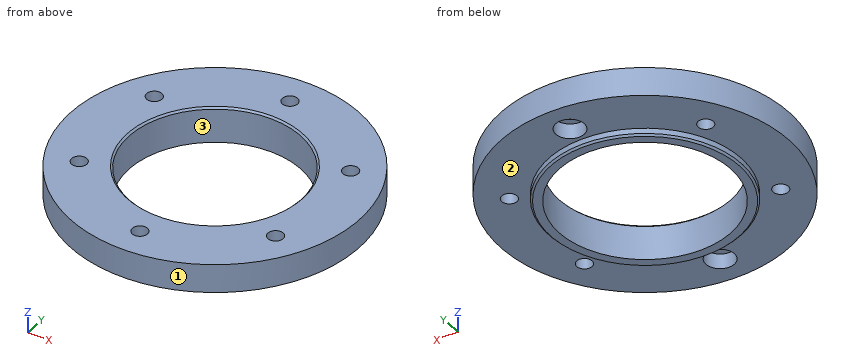
Autodesk Inventor part; units mm, degrees
ref_plane "YZ Plane" through (0, 0, 0) normal (1, 0, 0) x (0, 1, 0)
ref_plane "XZ Plane" through (0, 0, 0) normal (0, 1, 0) x (-1, 0, 0)
ref_plane "XY Plane" through (0, 0, 0) normal (0, 0, 1) x (1, 0, 0)
sketch "スケッチ2" plane through (0, 0, 0) normal (1, 0, 0) x (0, 1, 0)
  line L0 (24.1, 0) -> (24.1, -10)
  line L1 (40.5, 0) -> (40.5, -8)
  line L2 (40.5, 0) -> (24.1, 0)
  line L3 (24.1, 0) -> (59, 0)
  line L4 (24.1, -10) -> (27, -10)
  line L5 (0, -12) -> (0, 2)
  line L6 (27, -10) -> (27, -8)
  line L7 (27, -8) -> (40.5, -8)
  point P0 (0, 0)
  dimension "d40" = 24.1
  dimension "d41" = 8
  dimension "d42" = 40.5
  dimension "d43" = 27
  dimension "d44" = 2
revolve "回転1" add sketch "スケッチ2" angle 360 about axis through (0, 0, -10) along (0, 0, 1)
sketch "スケッチ4" plane through (0, 0, 0) normal (0, 0, 1) x (1, 0, 0)
  point P0 (0, 0)
  point P1 (0, 32)
  point P2 (-27.7128, 16)
  point P3 (-27.7128, -16)
  point P4 (0, -32)
  point P5 (27.7128, -16)
  point P6 (27.7128, 16)
  dimension "d11" = 32
  dimension "d14" = 360
hole "穴1" at (0, 32, 0) at (-27.7128, 16, 0) at (-27.7128, -16, 0) at (0, -32, 0) at (27.7128, -16, 0) at (27.7128, 16, 0) direction (0, 0, -1) diameter 4.3 end through all
chamfer "面取り3" distance 0.5 angle 45 1 edges at (0, -27, -10)
chamfer "面取り4" distance 0.5 angle 45 1 edges at (0, -24.1, 0)
sketch "スケッチ9" plane through (0, 0, -8) normal (0, 0, -1) x (-1, 0, 0)
  circle A0 centre (0, -32) radius 2.15
  circle A1 centre (0, 32) radius 2.15
  circle A2 centre (0, -32) radius 2.15
  circle A3 centre (0, -32) radius 4
  circle A4 centre (0, 32) radius 4
  point P0 (0, 0)
  dimension "d64" = 8
  dimension "d65" = 8
extrude "押し出し5" cut sketch "スケッチ9" against normal blind 4.2 contours A0 | A1 | A3 | A4
properties part number "scara-base1" material "ABS プラスチック"
Could you check a few things on this model? Use its own coordinates, in mm. Face numbers are marked on the shaded views. Round coordinates to 2 decimals unless told otherwise and drop trailing zeros. Write each loop counter-clockwise with the first axis right and the second up, starting at its lowest first coordinate (ties: lowest second). Pieces come first, ordered by that corner, then holes. Notation, with made-up numbers: M 39.5,6.5 L 85.5,6.5 A24 ccw 85.5,31.5 Z; hole C -3.75,34.25 d1. An arc over 180 degrees is marked long. Write each question's results on one line, items separated by ' | '. Start each with the question number.
1. Imagine slicing it at B-B on y = 0. List the corners of the cut face in (x, z) for me.
2. I need wall thicknesses on L1, parallel to Y at x = 0, z = -5.8; L2, parallel to Y at x = 0, z = -1.1; L3, parallel to X at y = 16, z = -4.5. Which ranges of each line are inside material? Lowest first, please. Write a range as from..to.
3. I'm going to push flat-ended pins straight in: pin 1 Ø2 at (y, z) = (-20, -1.5) entering from -X; pin 2 Ø7 at (x, y) = (-27.71, 16) entering from +Z; pin 3 Ø2.5 at (x, y) = (-27.71, -16) entering from +Z; pin 4 Ø9 at (x, y) = (-1.5, 32.5) entering from -Z. Where does each tip first touch, or does it pass through?
4. Thinking about a two-plate mould opening in X: for the marked faces 1, 2 and 3, which applies, +X half, -X half, draft (parallel to the pull), parting line (faces both ways), or undercut?
5. Imagine slicing it at D-D on y = 32. List the corners of the cut face in (x, z) for me, and give its area (3 significant figures).
6. Imagine slicing it at A-A on x = 0. Count the separate pieces of the cut face and the enclosed holes in it, and give its area (3 significant figures).
Result sheet:
1) outline: M -40.5,-8 L -27,-8 L -27,-9.5 L -26.5,-10 L -24.1,-10 L -24.1,-0.5 L -24.6,0 L -40.5,0 Z; M 24.1,-10 L 26.5,-10 L 27,-9.5 L 27,-8 L 40.5,-8 L 40.5,0 L 24.6,0 L 24.1,-0.5 Z
2) L1: y = -40.5..-36, -28..-24.1, 24.1..28, 36..40.5 | L2: y = -40.5..-34.15, -29.85..-24.1, 24.1..29.85, 34.15..40.5 | L3: x = -37.21..-29.86, -25.56..-18.02, 18.02..25.56, 29.86..37.21
3) pin 1: stops at x = -35.77 | pin 2: stops at z = 0 | pin 3: passes through | pin 4: stops at z = -8
4) face 1: parting line | face 2: draft | face 3: undercut
5) outline: M -24.82,-8 L -4,-8 L -4,-3.8 L -2.15,-3.8 L -2.15,0 L -24.82,0 Z; M 2.15,-3.8 L 4,-3.8 L 4,-8 L 24.82,-8 L 24.82,0 L 2.15,0 Z | area: 347 mm^2
6) separate pieces: 4 | enclosed holes: 0 | area: 174 mm^2
